Read the model definition and answer for the solid it produces. Units are mm, in the model's axes. A direction names the side the tool comes from. Coordinates: 2 decimals unless noted, no trailing zeros. Write each loop counter-clockwise with the first axis right and the second up, starting at its lowest first coordinate (ties: lowest second). Pieces come first, ordered by that corner, then holes.
(1) Section C-C on z = -552 is taken. Write down the section's boundary in (x, y), then the cut area to 3 significant figures.
(2) Which of the six approach directions +Z, -Z, +X, -X, +Y, -Y give full straight-line access (tool end or side, diameter ignored) to faces 1 (the flat face through (35, 75, -667)), 2 (the flat face through (35, 62, -44)), 3 (the flat face through (35, 39, -86)), 4 (the flat face through (35, 12, -710)), 5 (the flat face through (34.51, 59.252, -622.847))?
(3) The mould has two halves that part along Y. Classify faces 6 (the flat face through (35, 37, -145)), 7 (the flat face through (35, 25, -658)), 8 (the flat face through (0, 15, -350)): +Y half, -Y half, draft (parallel to the pull), parting line (faces both ways), or undercut.
(4) Given pin 1 (12 mm diameter, centred on x = 10, y = 57, fed in from -Z); pin 2 (6 mm diameter, centred on x = 31.5, y = 32.5, fed in from +Z); pin 3 (6 mm diameter, centred on x = 31.5, z = -436.5, fed in from +Y), each flat-ended and moving along its own axis, determine where each tip first touches the part or whether it passes through.
(5) Section A-A on z = -683 is taken. Write down the section's boundary in (x, y).
(6) Section B-B on x = 44 is taken. State how many separate pieces and enclosed holes the cut face has, then the cut area to 3 significant figures.
(7) Find the intervals of material crossed by probe 1 along Z at (x, y) = (35, 19); probe 2 along Z at (x, y) = (35, 53); probe 3 along Y at (x, z) = (32.5, -61.5), in increasing order.
from build123d import *

# Parameters (mm, degrees)
BOSS_EXTRUDE1_DEPTH = 70
SKETCH2_R           = 15
CUT_EXTRUDE1_DEPTH  = 88


with BuildPart() as part:
    # Sketch1 → Boss-Extrude1 (new body)
    with BuildSketch(Plane(origin=(0, 0, 0), x_dir=(0, 0, -1), z_dir=(1, 0, 0))):
        with BuildLine():
            ThreePointArc((94.142135624, 30.857864376), (100.6306026, 26.52240935), (108.284271247, 25))
            Line((108.284271247, 25), (0, 25))
            Line((0, 25), (0, 0))
            Line((0, 0), (710, 0))
            Line((710, 0), (710, 25))
            Line((710, 25), (605.381197846, 25))
            ThreePointArc((605.381197846, 25), (615.381197846, 27.679491924), (622.701705922, 35))
            Line((622.701705922, 35), (643.486315613, 71))
            ThreePointArc((643.486315613, 71), (646.414518843, 73.92820323), (650.414518843, 75))
            Line((650.414518843, 75), (710, 75))
            Line((710, 75), (710, 87))
            Line((710, 87), (650.414518843, 87))
            ThreePointArc((650.414518843, 87), (640.414518843, 84.320508076), (633.094010768, 77))
            Line((633.094010768, 77), (612.309401077, 41))
            ThreePointArc((612.309401077, 41), (609.381197846, 38.07179677), (605.381197846, 37))
            Line((605.381197846, 37), (570, 37))
            Line((570, 37), (570, 25))
            Line((570, 25), (180, 25))
            Line((180, 25), (180, 37))
            Line((180, 37), (108.313708499, 37))
            ThreePointArc((108.313708499, 37), (105.25224104, 37.60896374), (102.656854249, 39.343145751))
            Line((102.656854249, 39.343145751), (85.857864376, 56.142135624))
            ThreePointArc((85.857864376, 56.142135624), (79.3693974, 60.47759065), (71.715728753, 62))
            Line((71.715728753, 62), (0, 62))
            Line((0, 62), (0, 50))
            Line((0, 50), (71.686291501, 50))
            ThreePointArc((71.686291501, 50), (74.74775896, 49.39103626), (77.343145751, 47.656854249))
            Line((77.343145751, 47.656854249), (94.142135624, 30.857864376))
        make_face()
    extrude(amount=BOSS_EXTRUDE1_DEPTH)

    # Sketch2 → Cut-Extrude1 (cut, through all)
    with BuildSketch(Plane(origin=(0, 0, 0), x_dir=(1, 0, 0), z_dir=(0, 1, 0))):
        with Locations((35, 683)):
            Circle(SKETCH2_R)
        with Locations((35, 27)):
            Circle(SKETCH2_R)
    extrude(amount=CUT_EXTRUDE1_DEPTH, mode=Mode.SUBTRACT)


solid = part.part
Response:
1. outline: (0, 0) - (70, 0) - (70, 25) - (0, 25) - close
1. area: 1,750 mm2
2. face 1: -Z, +X, -X
2. face 2: +Z, +X, -X, +Y
2. face 3: +Z, +X, -X
2. face 4: -Z, +X, -X, +Y, -Y
2. face 5: +X, -X, +Y
3. face 6: +Y half
3. face 7: undercut
3. face 8: draft
4. pin 1: stops at z = -638.87
4. pin 2: stops at z = -89.5
4. pin 3: stops at y = 25
5. outline: (0, 0) - (20, 0) - (20, 25) - (0, 25) - close; (0, 75) - (20, 75) - (20, 87) - (0, 87) - close; (50, 0) - (70, 0) - (70, 25) - (50, 25) - close; (50, 75) - (70, 75) - (70, 87) - (50, 87) - close
6. separate pieces: 5
6. enclosed holes: 0
6. area: 20,200 mm2
7. probe 1: z = -710 to -698, -668 to -42, -12 to 0
7. probe 2: z = -633.09 to -619.24, -89 to -42, -12 to 0
7. probe 3: y = 0 to 25, 50 to 62
